Read the model definition and answer for the solid it produces. Units are mm, in the model's axes. Face numbers are marked on the shaded views. Round coordinates to 2 decimals unless told otherwise and drop trailing zeros. Loops run counter-clockwise (first coordinate to the right, second up) from the corner with the lowest first, then second, coordinate; pieces in that order, holes last. Notation, with made-up numbers: (-1.75, -4) - (14.25, -4) arc R22 ccw to (14.25, 17) - close; hole circle Ø11 at (30.25, -34). An arc over 180 degrees is marked (long way). Use one line per item in the form item = value. Start each with the question number.
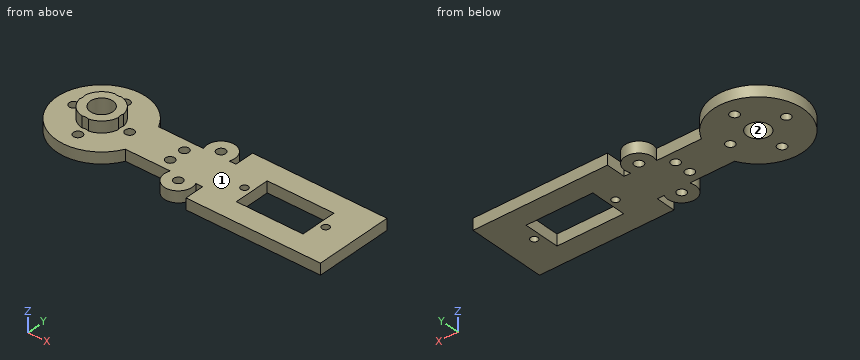
```python
from build123d import *

# Parameters (mm, degrees)
MAIN_WEB_PROFILE_W                        = 60
MAIN_WEB_PROFILE_H                        = 14
MAIN_WEB_DEPTH                            = 4
SHOULDER_HORN_FLANGE_PROFILE_R            = 16
SHOULDER_HORN_FLANGE_DEPTH                = 4
ELBOW_SERVO_MOUNT_PROFILE_W               = 48
ELBOW_SERVO_MOUNT_PROFILE_H               = 28
ELBOW_SERVO_MOUNT_DEPTH                   = 4
SG90_BODY_CLEARANCE_START                 = -5
SG90_BODY_CLEARANCE_PROFILE_W             = 23.8
SG90_BODY_CLEARANCE_PROFILE_H             = 13
SG90_BODY_CLEARANCE_DEPTH                 = 97.49863387
ELBOW_TAB_FASTENERS_START                 = -50
ELBOW_TAB_FASTENERS_PROFILE_R             = 1.3
ELBOW_TAB_FASTENERS_DEPTH                 = 142.49863387
SHOULDER_CENTER_SCREW_ACCESS_START        = -50
SHOULDER_CENTER_SCREW_ACCESS_PROFILE_R    = 4
SHOULDER_CENTER_SCREW_ACCESS_DEPTH        = 142.49863387
SHOULDER_HORN_BOLT_PATTERN_START          = -50
SHOULDER_HORN_BOLT_PATTERN_PROFILE_R      = 1.6
SHOULDER_HORN_BOLT_PATTERN_DEPTH          = 142.49863387
CABLE_TIE_HOLES_START                     = -50
CABLE_TIE_HOLES_PROFILE_R                 = 1.6
CABLE_TIE_HOLES_DEPTH                     = 142.49863387
PASSIVE_LOWER_MOUNT_BOSS_PROFILE_R        = 5
PASSIVE_LOWER_MOUNT_BOSS_DEPTH            = 4
PASSIVE_UPPER_MOUNT_BOSS_PROFILE_R        = 5
PASSIVE_UPPER_MOUNT_BOSS_DEPTH            = 4
PASSIVE_CHEEK_STANDOFFS_START             = -50
PASSIVE_CHEEK_STANDOFFS_PROFILE_R         = 1.6
PASSIVE_CHEEK_STANDOFFS_DEPTH             = 142.49863387
SHOULDER_DOWEL_SUPPORT_HUB_START          = 4
SHOULDER_DOWEL_SUPPORT_HUB_PROFILE_R      = 7
SHOULDER_DOWEL_SUPPORT_HUB_PROFILE_R_2    = 4
SHOULDER_DOWEL_SUPPORT_HUB_DEPTH          = 4
SHOULDER_HORN_WASHER_HUB_RELIEF_START     = 4
SHOULDER_HORN_WASHER_HUB_RELIEF_PROFILE_R = 3.3
SHOULDER_HORN_WASHER_HUB_RELIEF_DEPTH     = 4


with BuildPart() as part:
    # Main_web_profile → Main_web (new body)
    with BuildSketch(Plane.XY):
        with Locations((30, 0)):
            Rectangle(MAIN_WEB_PROFILE_W, MAIN_WEB_PROFILE_H)
    extrude(amount=MAIN_WEB_DEPTH)

    # Shoulder_horn_flange_profile → Shoulder_horn_flange (add)
    with BuildSketch(Plane.XY):
        Circle(SHOULDER_HORN_FLANGE_PROFILE_R)
    extrude(amount=SHOULDER_HORN_FLANGE_DEPTH)

    # Elbow_servo_mount_profile → Elbow_servo_mount (add)
    with BuildSketch(Plane.XY):
        with Locations((66, 0)):
            Rectangle(ELBOW_SERVO_MOUNT_PROFILE_W, ELBOW_SERVO_MOUNT_PROFILE_H)
    extrude(amount=ELBOW_SERVO_MOUNT_DEPTH)

    # SG90_body_clearance_profile → SG90_body_clearance (cut, through all)
    with BuildSketch(Plane.XY.offset(SG90_BODY_CLEARANCE_START)):
        with Locations((65.5, 0)):
            Rectangle(SG90_BODY_CLEARANCE_PROFILE_W, SG90_BODY_CLEARANCE_PROFILE_H)
    extrude(amount=SG90_BODY_CLEARANCE_DEPTH, mode=Mode.SUBTRACT)

    # Elbow_tab_fasteners_profile → Elbow_tab_fasteners (cut, through all)
    with BuildSketch(Plane.XY.offset(ELBOW_TAB_FASTENERS_START)):
        with Locations(Location((51, 0, 0), (0, 0, 180))):
            Circle(ELBOW_TAB_FASTENERS_PROFILE_R)
        with Locations(Location((80, 0, 0), (0, 0, 180))):
            Circle(ELBOW_TAB_FASTENERS_PROFILE_R)
    extrude(amount=ELBOW_TAB_FASTENERS_DEPTH, mode=Mode.SUBTRACT)

    # Shoulder_center_screw_access_profile → Shoulder_center_screw_access (cut, through all)
    with BuildSketch(Plane.XY.offset(SHOULDER_CENTER_SCREW_ACCESS_START)):
        with Locations(Location((0, 0, 0), (0, 0, 180))):
            Circle(SHOULDER_CENTER_SCREW_ACCESS_PROFILE_R)
    extrude(amount=SHOULDER_CENTER_SCREW_ACCESS_DEPTH, mode=Mode.SUBTRACT)

    # Shoulder_horn_bolt_pattern_profile → Shoulder_horn_bolt_pattern (cut, through all)
    with BuildSketch(Plane.XY.offset(SHOULDER_HORN_BOLT_PATTERN_START)):
        with Locations(Location((0, 10, 0), (0, 0, 180))):
            Circle(SHOULDER_HORN_BOLT_PATTERN_PROFILE_R)
        with Locations(Location((0, -10, 0), (0, 0, 180))):
            Circle(SHOULDER_HORN_BOLT_PATTERN_PROFILE_R)
        with Locations(Location((10, 0, 0), (0, 0, 180))):
            Circle(SHOULDER_HORN_BOLT_PATTERN_PROFILE_R)
        with Locations(Location((-10, 0, 0), (0, 0, 180))):
            Circle(SHOULDER_HORN_BOLT_PATTERN_PROFILE_R)
    extrude(amount=SHOULDER_HORN_BOLT_PATTERN_DEPTH, mode=Mode.SUBTRACT)

    # Cable_tie_holes_profile → Cable_tie_holes (cut, through all)
    with BuildSketch(Plane.XY.offset(CABLE_TIE_HOLES_START)):
        with Locations(Location((27, -3, 0), (0, 0, 180))):
            Circle(CABLE_TIE_HOLES_PROFILE_R)
        with Locations(Location((27, 3, 0), (0, 0, 180))):
            Circle(CABLE_TIE_HOLES_PROFILE_R)
    extrude(amount=CABLE_TIE_HOLES_DEPTH, mode=Mode.SUBTRACT)

    # Passive_lower_mount_boss_profile → Passive_lower_mount_boss (add)
    with BuildSketch(Plane.XY):
        with Locations((35, -9)):
            Circle(PASSIVE_LOWER_MOUNT_BOSS_PROFILE_R)
    extrude(amount=PASSIVE_LOWER_MOUNT_BOSS_DEPTH)

    # Passive_upper_mount_boss_profile → Passive_upper_mount_boss (add)
    with BuildSketch(Plane.XY):
        with Locations((35, 9)):
            Circle(PASSIVE_UPPER_MOUNT_BOSS_PROFILE_R)
    extrude(amount=PASSIVE_UPPER_MOUNT_BOSS_DEPTH)

    # Passive_cheek_standoffs_profile → Passive_cheek_standoffs (cut, through all)
    with BuildSketch(Plane.XY.offset(PASSIVE_CHEEK_STANDOFFS_START)):
        with Locations(Location((35, -9, 0), (0, 0, 180))):
            Circle(PASSIVE_CHEEK_STANDOFFS_PROFILE_R)
        with Locations(Location((35, 9, 0), (0, 0, 180))):
            Circle(PASSIVE_CHEEK_STANDOFFS_PROFILE_R)
    extrude(amount=PASSIVE_CHEEK_STANDOFFS_DEPTH, mode=Mode.SUBTRACT)

    # Shoulder_dowel_support_hub_profile → Shoulder_dowel_support_hub (add)
    with BuildSketch(Plane.XY.offset(SHOULDER_DOWEL_SUPPORT_HUB_START)):
        Circle(SHOULDER_DOWEL_SUPPORT_HUB_PROFILE_R)
        with Locations(Location((0, 0, 0), (0, 0, 180))):
            Circle(SHOULDER_DOWEL_SUPPORT_HUB_PROFILE_R_2, mode=Mode.SUBTRACT)
    extrude(amount=SHOULDER_DOWEL_SUPPORT_HUB_DEPTH)

    # Shoulder_horn_washer_hub_relief_profile → Shoulder_horn_washer_hub_relief (cut)
    with BuildSketch(Plane.XY.offset(SHOULDER_HORN_WASHER_HUB_RELIEF_START)):
        with Locations((10, 0)):
            Circle(SHOULDER_HORN_WASHER_HUB_RELIEF_PROFILE_R)
        with Locations((-10, 0)):
            Circle(SHOULDER_HORN_WASHER_HUB_RELIEF_PROFILE_R)
        with Locations((0, 10)):
            Circle(SHOULDER_HORN_WASHER_HUB_RELIEF_PROFILE_R)
        with Locations((0, -10)):
            Circle(SHOULDER_HORN_WASHER_HUB_RELIEF_PROFILE_R)
    extrude(amount=SHOULDER_HORN_WASHER_HUB_RELIEF_DEPTH, mode=Mode.SUBTRACT)


solid = part.part
```
1) Determine the mould class of the marked faces 1 and 2 for opening direction Y: +Y half, -Y half, draft (parallel to the pull), parting line (faces both ways), or undercut.
2) A cutting plane is placed at C-C on y = 0. Count the separate pieces of the cut face and the enclosed holes in it, plus the area to 3 significant figures.
3) Straight lines are drawn through the part: line 1 (Y direction, x = 35, z = 1.65); line 2 (Y direction, x = 0, z = 1.7); line 3 (Y direction, x = 0.5, z = 3). For each, find the intervals that lie inside material, in ascending order. Write a range as from..to.
4) A cutting plane is placed at B-B on z = 7. Write down the section's boundary in (x, y).
5) A cutting plane is placed at A-A on x = 51. Write down the section's boundary in (y, z), plus the area to 3 significant figures.
6) Flat-ended cylindrical pins translate along their axes: pin 1 (3 mm diameter, centred on x = 62.5, z = 2, fed in from +Y); pin 2 (1.5 mm diameter, centred on x = 34, y = 10.5, fed in from +Z); pin 3 (2 mm diameter, centred on x = 51, y = 0, fed in from +Z); pin 4 (1.9 mm diameter, centred on x = 40.5, z = 1.5, fed in from +Y). Find the tip coordinate at first contact, or state that the pin passes through.
Checks:
q1.face_1 = draft
q1.face_2 = undercut
q2.separate_pieces = 7
q2.enclosed_holes = 0
q2.area = 272 mm²
q3.line_1 = -14..-10.6, -7.4..7.4, 10.6..14
q3.line_2 = -16..-11.6, -8.4..-4, 4..8.4, 11.6..16
q3.line_3 = -15.99..-11.52, -8.48..-3.97, 3.97..8.48, 11.52..15.99
q4.outline = (-6.91, -1.15) arc R7 ccw to (-1.15, -6.91) arc R3.3 cw to (1.15, -6.91) arc R7 ccw to (6.91, -1.15) arc R3.3 cw to (6.91, 1.15) arc R7 ccw to (1.15, 6.91) arc R3.3 cw to (-1.15, 6.91) arc R7 ccw to (-6.91, 1.15) arc R3.3 cw to start; hole circle Ø8 at (0, 0)
q5.outline = (-14, 0) - (-1.3, 0) - (-1.3, 4) - (-14, 4) - close; (1.3, 0) - (14, 0) - (14, 4) - (1.3, 4) - close
q5.area = 102 mm²
q6.pin_1 = 14
q6.pin_2 = 4
q6.pin_3 = through
q6.pin_4 = 11.07
